Source: CAD feature listing. Evaluate the final solid. Frame: model axes, mm. A direction names the side the tool comes from. Give positions to 0.01 mm unless a question says otherwise; leave off trailing zeros. Order: outer loops, then holes, each group sorted by start corner. A loop starts at its lowest first (then second) coordinate and runs counter-clockwise, first axis right, second up.
from build123d import *

# Parameters (mm, degrees)
SKETCH1_R           = 4.5
SKETCH1_R_2         = 1.15
BOSS_EXTRUDE1_DEPTH = 5.08
SKETCH4_W           = 23
SKETCH4_H           = 15
CUT_EXTRUDE1_DEPTH  = 1


with BuildPart() as part:
    # Sketch1 → Boss-Extrude1 (new body)
    with BuildSketch(Plane(origin=(0, 0, 0), x_dir=(1, 0, 0), z_dir=(0, 1, 0))):
        Polygon((-14, 8.77), (12.77, 8.77), (12.77, -18.1), (5.735, -18.1), (5.735, -15.56), (-6.965, -15.56), (-6.965, -18.1), (-14, -18.1), align=None)
        with Locations(Location((-5.715, 0, 0), (0, 0, 270))):
            Circle(SKETCH1_R, mode=Mode.SUBTRACT)
        with Locations(Location((5.715, 0, 0), (0, 0, 270))):
            Circle(SKETCH1_R, mode=Mode.SUBTRACT)
        with Locations(Location((-9.384999986, -9.8, 0), (0, 0, 270))):
            Circle(SKETCH1_R_2, mode=Mode.SUBTRACT)
        with Locations(Location((8.154999986, -9.8, 0), (0, 0, 270))):
            Circle(SKETCH1_R_2, mode=Mode.SUBTRACT)
    extrude(amount=BOSS_EXTRUDE1_DEPTH)

    # Sketch4 → Cut-Extrude1 (cut)
    with BuildSketch(Plane(origin=(0, 5.08, 0), x_dir=(1, 0, 0), z_dir=(0, 1, 0))):
        Rectangle(SKETCH4_W, SKETCH4_H)
    extrude(amount=-CUT_EXTRUDE1_DEPTH, mode=Mode.SUBTRACT)


solid = part.part
(1) Section A-A, the plane z = 9.8. Return loops of the section in (x, y) (3 decimals).
(2) Line query: line 1 along X through (y, z) = (2.2, 9.8) (3 decimals); line 2 along X through (y, z) = (2.3, 0) (3 decimals); line 3 along X through (y, z) = (4.55, 0.5). Output: solid intervals per line, ascending.
(3) Section C-C, the plane z = 6. Return loops of the section in (x, y), plus the area to 3 significant figures.
(4) Draft query along Z for faces 4 (the flat face through (-1, 3, -8.77)), 5 (the flat face through (-11.5, 4.6, 0.1)), 6 (the flat face through (-1, 5.08, 10)), 7 (the cylindrical face through (-9.04, 2.504, 10.897)). Return one class per face: +Z half, -Z half, draft (parallel to the pull), parting line (faces both ways), or undercut.
(5) Access query for faces 1 (the flat face through (12.77, 3, 4)), 2 (the flat face through (11.5, 4.6, 0.1)), 3 (the flat face through (5.735, 3, 17)). Directions: +Z, -Z, +X, -X, +Y, -Y. A direction counts if a zero-diameter tool reaches every point of the face in a straight line with its end or side. Return the directions, or none.
(6) Section B-B, the plane x = 4. Return loops of the section in (y, z), plus the area to 3 significant figures.
(7) Pin query (flat end, axial travel): pin 1 Ø2.5 at (x, z) = (8.155, 9.8) entering from +Y; pin 2 Ø7 at (x, z) = (-5.715, 0) entering from -Y; pin 3 Ø4.5 at (x, z) = (-3, -0.5) entering from +Y; pin 4 Ø2.5 at (x, y) = (2, 1.5) entering from +Z. Return the tip coordinate at first contact, or that it passes through.
(8) Section D-D, the plane x = -9.75. Return loops of the section in (y, z), plus the area to 3 significant figures.
Checks:
1. outline: (-14, 0) - (-10.535, 0) - (-10.535, 5.08) - (-14, 5.08) - close; (-8.235, 0) - (7.005, 0) - (7.005, 5.08) - (-8.235, 5.08) - close; (9.305, 0) - (12.77, 0) - (12.77, 5.08) - (9.305, 5.08) - close
2. line 1: x = -14 to -10.535, -8.235 to 7.005, 9.305 to 12.77
2. line 2: x = -14 to -10.215, -1.215 to 1.215, 10.215 to 12.77
2. line 3: x = -14 to -11.5, 11.5 to 12.77
3. outline: (-14, 0) - (12.77, 0) - (12.77, 5.08) - (11.5, 5.08) - (11.5, 4.08) - (-11.5, 4.08) - (-11.5, 5.08) - (-14, 5.08) - close
3. area: 113 mm2
4. face 4: -Z half
4. face 5: undercut
4. face 6: draft
4. face 7: undercut
5. face 1: +Z, -Z, +X, +Y, -Y
5. face 2: +Y
5. face 3: +Z, +Y, -Y
6. outline: (0, -8.77) - (5.08, -8.77) - (5.08, -7.5) - (4.08, -7.5) - (4.08, -4.16) - (0, -4.16) - close; (0, 4.16) - (4.08, 4.16) - (4.08, 7.5) - (5.08, 7.5) - (5.08, 15.56) - (0, 15.56) - close
6. area: 74.6 mm2
7. pin 1: stops at y = 5.08
7. pin 2: passes through
7. pin 3: stops at y = 4.08
7. pin 4: stops at z = 15.56
8. outline: (0, -8.77) - (5.08, -8.77) - (5.08, -7.5) - (4.08, -7.5) - (4.08, -1.99) - (0, -1.99) - close; (0, 1.99) - (4.08, 1.99) - (4.08, 7.5) - (5.08, 7.5) - (5.08, 8.71) - (0, 8.71) - close; (0, 10.89) - (5.08, 10.89) - (5.08, 18.1) - (0, 18.1) - close
8. area: 94.2 mm2
